```python
from build123d import *

# Parameters (mm, degrees)
F4_DEPTH  = 20
F5_W      = 3.4
F5_H      = 20.6
F5_W_2    = 20.6
F5_H_2    = 3.4
F5_W_3    = 18.6
F5_H_3    = 18.6
F6_DEPTH  = 2
F7_DEPTH  = 2
F8_W      = 20.6
F8_H      = 9.4
F9_DEPTH  = 3.4
F10_W     = 30
F10_H     = 30
F11_DEPTH = 4
F12_R     = 5


with BuildPart() as f4:
    # F3 (on Top) → F4 (new body)
    with BuildSketch(Plane.XY):
        Polygon((0, 18.6), (-4, 18.6), (-4, -2), (-7.4, -2), (-7.4, 18.6), (-11.4, 18.6), (-11.4, -11.4), (18.6, -11.4), (18.6, -7.4), (-2, -7.4), (-2, -4), (18.6, -4), (18.6, 0), (0, 0), align=None)
    extrude(amount=F4_DEPTH)

    # F5 (on face) → F6 (join)
    with BuildSketch(Plane.XY.offset(20)):
        with Locations((-5.7, 8.3)):
            Rectangle(F5_W, F5_H)
        Polygon((-11.4, 18.6), (-11.4, -11.4), (18.6, -11.4), (18.6, -7.4), (-2, -7.4), (-2, -4), (18.6, -4), (18.6, 0), (0, 0), (0, 18.6), (-4, 18.6), (-4, -2), (-7.4, -2), (-7.4, 18.6), align=None)
        with Locations((8.3, -5.7)):
            Rectangle(F5_W_2, F5_H_2)
        with Locations((9.3, 9.3)):
            Rectangle(F5_W_3, F5_H_3)
    extrude(amount=F6_DEPTH)

    # F7 (add): a face of the model
    f7_faces = [f4.faces().sort_by_distance(p)[0] for p in [
        (3.6, 3.6, 22),
    ]]
    extrude(f7_faces, amount=F7_DEPTH)

    # F8 (on face) → F9 (join)
    with BuildSketch(Plane.XY.offset(24)):
        Polygon((-2, 18.6), (-11.4, 18.6), (-11.4, -11.4), (-2, -11.4), (-2, -2), align=None)
        with Locations((8.3, -6.7)):
            Rectangle(F8_W, F8_H)
    extrude(amount=F9_DEPTH)

    # F10 (on face) → F11 (join)
    with BuildSketch(Plane.XY.offset(27.4)):
        with Locations((3.6, 3.6)):
            Rectangle(F10_W, F10_H)
    extrude(amount=F11_DEPTH)

    # F12
    f12_edges = [f4.edges().sort_by_distance(p)[0] for p in [
        (0, 0, 10),
        (0, 9.3, 20),
        (9.3, 0, 20),
    ]]
    fillet(f12_edges, radius=F12_R)


solid = f4.part
```
Read the model definition and answer for the solid it produces. Units are mm, in the model's axes. A direction names the side the tool comes from. Give positions to 0.01 mm unless a question says otherwise; leave off trailing zeros. Write each loop counter-clockwise with the first axis right and the second up, starting at its lowest first coordinate (ties: lowest second). Pieces come first, ordered by that corner, then holes. Notation, with made-up numbers: (-9.75, -36) - (-0.75, -36) arc R20 ccw to (-0.75, 1) - close; hole circle Ø3 at (37, 25.25). An arc over 180 degrees is marked (long way). Write item = value, one per line. Start each with the question number.
Item 1: Each of these flat-tipped pins is pushed along its axis until it touches: P1, Ø11, axis at x = 13.5, y = 13.5, coming from the -Z side; P2, Ø3.5, axis at x = -5, z = 15, coming from the +Y side; P3, Ø2, axis at x = 14, y = 1.5, coming from the -Z side; P4, Ø16, axis at x = 11, z = 6, coming from the +Y side. Where does it stop, or does it pass through?
Item 2: Find section D-D (z = 24.5). Give the vertices of the cut face in (x, y).
Item 3: Find section A-A (x = -1.5). Give the vertices of the cut face in (y, z), then the cut area to 3 significant figures.
Item 4: Find section B-B (y = 1). Give the vertices of the cut face in (x, z).
Item 5: The mould has two halves that part along Z. Classify faces 1 (the flat face through (-2, 8, 26)), 2 (the flat face through (8, -6, 20)), 3 (the flat face through (12, 0, 7)): +Z half, -Z half, draft (parallel to the pull), parting line (faces both ways), or undercut.
Item 6: Find section C-C (z = 18). Give the vertices of the cut face in (x, y).
Item 7: A tool of negligible diameter and unlimited length cuts with its end or side. For faces 4 (the flat face through (-7.4, 8, 10)), 5 (the cylindrical face through (1, 12, 18)), 6 (the flat face through (8, -2, 26)), from which of +Z, -Z, +X, -X, +Y, -Y can it reach the whole face along a straight path? Write none if from no direction.
Item 8: Find the intervals of material crossed by probe 1 along Z at (x, y) = (16.5, 17.25); probe 2 along Y at (x, z) = (11.25, 8); probe 3 along Z at (x, y) = (-1, -1.5), in increasing order. Write a range as [from, to].
Response:
q1.P1 = 20
q1.P2 = 18.6
q1.P3 = 17.18
q1.P4 = 0.42
q2.outline = (-11.4, -11.4) - (18.6, -11.4) - (18.6, -2) - (-2, -2) - (-2, 18.6) - (-11.4, 18.6) - close
q3.outline = (-11.4, 0) - (-7.4, 0) - (-7.4, 20) - (-4, 20) - (-4, 0) - (18.6, 0) - (18.6, 24) - (-2, 24) - (-2, 27.4) - (18.6, 27.4) - (18.6, 31.4) - (-11.4, 31.4) - close
q3.area = 804 mm²
q4.outline = (-11.4, 0) - (-7.4, 0) - (-7.4, 20) - (-4, 20) - (-4, 0) - (2, 0) - (2, 15) arc R3 cw to (5, 18) - (18.6, 18) - (18.6, 24) - (-2, 24) - (-2, 27.4) - (18.6, 27.4) - (18.6, 31.4) - (-11.4, 31.4) - close
q5.face_1 = undercut
q5.face_2 = -Z half
q5.face_3 = draft
q6.outline = (-11.4, -11.4) - (18.6, -11.4) - (18.6, -7.4) - (-2, -7.4) - (-2, -4) - (18.6, -4) - (18.6, 1) - (5, 1) arc R4 cw to (1, 5) - (1, 18.6) - (-4, 18.6) - (-4, -2) - (-7.4, -2) - (-7.4, 18.6) - (-11.4, 18.6) - close
q7.face_4 = -Z, +Y
q7.face_5 = -Z, +X, +Y
q7.face_6 = +X, +Y
q8.probe_1 = [20, 24], [27.4, 31.4]
q8.probe_2 = [-11.4, -7.4], [-4, 0]
q8.probe_3 = [0, 24], [27.4, 31.4]
